Could you check a few things on this model? Use its own coordinates, in mm. Face numbers are marked on the shaded views. A direction names the side the tool comes from. Coordinates: 2 decimals unless noted, no trailing zeros. Write each loop counter-clockwise with the first axis right and the second up, starting at its lowest first coordinate (ties: lowest second). Pieces come first, ordered by that corner, then holes.
Item 1: I want a section at C-C on z = 3. Please give me the cut outline in (x, y).
Item 2: Which directions (+Z, -Z, +X, -X, +Y, -Y) give clear straight access to the entire face, cutting with the end or side of a thin tool? Please do the marked faces 5, 6 and 7.
Item 3: If I drill on probe 1 along X at (y, z) = (2, 10); probe 2 along X at (y, z) = (10, -14); probe 3 along X at (y, z) = (8, -11.5), over which ranges is the centre line in solid material (lowest first)?
Item 4: I want a section at A-A on x = 34.5. Please give me the cut outline in (y, z).
Item 5: Thinking about a two-plate mould opening in X: for the marked faces 1, 2, 3 and 4, which applies, +X half, -X half, draft (parallel to the pull), parting line (faces both ways), or undercut?
Item 6: For P1, Ø7, axis at x = 31.6, y = 4, coming from the -Z side, with a flat end and sliding along its axis, tell me the tip position at first contact or that it passes through.
Item 7: I want a section at B-B on z = -7. Please give me the cut outline in (x, y).
Item 8: I want a section at D-D on x = 6. Please give me the cut outline in (y, z).
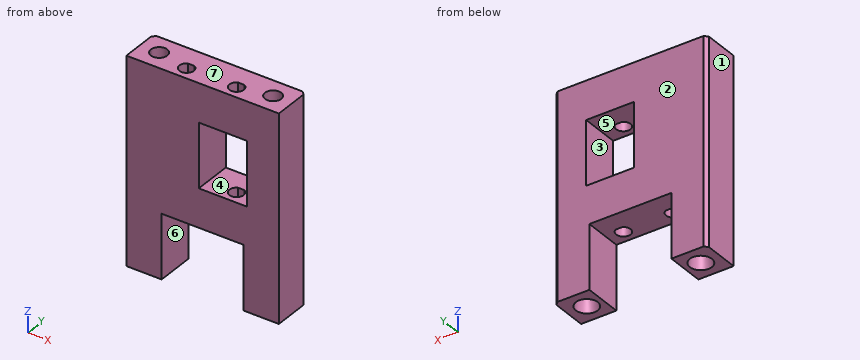
from build123d import *
from OCP.BRepFilletAPI import BRepFilletAPI_MakeChamfer

# Parameters (mm, degrees)
BOSS_EXTRUDE1_DEPTH = 44
SKETCH2_R           = 2.25
CUT_EXTRUDE1_DEPTH  = 66.098079849
BOSS_EXTRUDE2_START = 20
BOSS_EXTRUDE2_DEPTH = 20
BOSS_EXTRUDE3_START = -64
BOSS_EXTRUDE3_DEPTH = 64
SKETCH6_W           = 25.6
SKETCH6_H           = 20
CUT_EXTRUDE2_DEPTH  = 66.098079849
CHAMFER1_SIZE       = 10
CHAMFER1_SIZE2      = 0.874886635
CHAMFER2_SIZE       = 1
SKETCH7_W           = 15
SKETCH7_H           = 20
CUT_EXTRUDE3_DEPTH  = 66.922378598


with BuildPart() as part:
    # Sketch1 → Boss-Extrude1 (new body)
    with BuildSketch(Plane.XY):
        with BuildLine():
            Line((0, 0), (47.6, 0))
            Line((47.6, 0), (47.6, 6))
            Line((47.6, 6), (44.15, 6))
            ThreePointArc((44.15, 6), (41.6, 3.45), (39.05, 6))
            Line((39.05, 6), (8.55, 6))
            ThreePointArc((8.55, 6), (6, 3.45), (3.45, 6))
            Line((3.45, 6), (0, 6))
            Line((0, 6), (0, 0))
        make_face()
    extrude(amount=BOSS_EXTRUDE1_DEPTH)

    # Sketch2 → Cut-Extrude1 (cut, through all)
    with BuildSketch(Plane.XY.offset(44)):
        with Locations((16, 4)):
            Circle(SKETCH2_R)
        with Locations((31.6, 4)):
            Circle(SKETCH2_R)
    extrude(amount=-CUT_EXTRUDE1_DEPTH, mode=Mode.SUBTRACT)

    # Sketch4 → Boss-Extrude2 (add)
    with BuildSketch(Plane(origin=(0, 0, 0), x_dir=(-1, 0, 0), z_dir=(0, 0, -1)).offset(BOSS_EXTRUDE2_START)):
        with BuildLine():
            Line((-11, 6), (-11, 0))
            Line((-11, 0), (0, 0))
            Line((0, 0), (0, 6))
            Line((0, 6), (-3.45, 6))
            ThreePointArc((-3.45, 6), (-6, 3.45), (-8.55, 6))
            Line((-8.55, 6), (-11, 6))
        make_face()
        with BuildLine():
            Line((-36.6, 6), (-36.6, 0))
            Line((-36.6, 0), (-47.6, 0))
            Line((-47.6, 0), (-47.6, 6))
            Line((-47.6, 6), (-44.15, 6))
            ThreePointArc((-44.15, 6), (-41.6, 3.45), (-39.05, 6))
            Line((-39.05, 6), (-36.6, 6))
        make_face()
    extrude(amount=-BOSS_EXTRUDE2_DEPTH)

    # Sketch5 → Boss-Extrude3 (add)
    with BuildSketch(Plane.XY.offset(44).offset(BOSS_EXTRUDE3_START)):
        with BuildLine():
            Line((0, 6), (0, 12))
            Line((0, 12), (47.6, 12))
            Line((47.6, 12), (47.6, 6))
            Line((47.6, 6), (44.15, 6))
            ThreePointArc((44.15, 6), (41.6, 8.55), (39.05, 6))
            Line((39.05, 6), (8.55, 6))
            ThreePointArc((8.55, 6), (6, 8.55), (3.45, 6))
            Line((3.45, 6), (0, 6))
        make_face()
    extrude(amount=BOSS_EXTRUDE3_DEPTH)

    # Sketch6 → Cut-Extrude2 (cut, through all)
    with BuildSketch(Plane.XZ.offset(-6)):
        with Locations((23.8, -10)):
            Rectangle(SKETCH6_W, SKETCH6_H)
    extrude(amount=-CUT_EXTRUDE2_DEPTH, mode=Mode.SUBTRACT)

    # Chamfer1: one chamfer whose edges measure the first distance from different faces: ONE call of the kernel's chamfer builder (chamfer() names one face for all edges)
    chamfer1_edges_1 = [part.edges().sort_by_distance(p)[0] for p in [
        (6, 3.45, -20),
    ]]
    chamfer1_side_1 = [part.faces().sort_by_distance(p)[0] for p in [
        (6, 3.45, 12),
    ]]
    chamfer1_edges_2 = [part.edges().sort_by_distance(p)[0] for p in [
        (41.6, 8.55, -20),
    ]]
    chamfer1_side_2 = [part.faces().sort_by_distance(p)[0] for p in [
        (41.6, 8.55, 12),
    ]]
    chamfer1 = BRepFilletAPI_MakeChamfer(part.part.solid().wrapped)
    for e in chamfer1_edges_1:
        chamfer1.Add(CHAMFER1_SIZE, CHAMFER1_SIZE2, e.wrapped, chamfer1_side_1[0].wrapped)  # the first distance lies on this face
    for e in chamfer1_edges_2:
        chamfer1.Add(CHAMFER1_SIZE, CHAMFER1_SIZE2, e.wrapped, chamfer1_side_2[0].wrapped)  # the first distance lies on this face
    add(Compound.cast(chamfer1.Shape()), mode=Mode.REPLACE)

    # Chamfer2
    chamfer2_edges = [part.edges().sort_by_distance(p)[0] for p in [
        (47.6, 12, 12),
        (0, 12, 12),
    ]]
    chamfer(chamfer2_edges, length=CHAMFER2_SIZE)

    # Sketch7 → Cut-Extrude3 (cut, through all)
    with BuildSketch(Plane.XZ):
        with Locations((30.1, 22)):
            Rectangle(SKETCH7_W, SKETCH7_H)
    extrude(amount=-CUT_EXTRUDE3_DEPTH, mode=Mode.SUBTRACT)


solid = part.part
Response values:
1. outline: (0, 0) - (47.6, 0) - (47.6, 11) - (46.6, 12) - (1, 12) - (0, 11) - close; hole circle Ø5.1 at (6, 6); hole (14.97, 6) arc R2.25 ccw (long way) to (17.03, 6) - close; hole (30.57, 6) arc R2.25 ccw (long way) to (32.63, 6) - close; hole circle Ø5.1 at (41.6, 6)
2. face 5: +Y, -Y
2. face 6: -Z, +Y, -Y
2. face 7: +Z, +X, -X, +Y, -Y
3. probe 1: x = 0 to 14.97, 17.03 to 30.57, 32.63 to 47.6
3. probe 2: x = 0 to 11, 36.6 to 47.6
3. probe 3: x = 0 to 4.21, 7.79 to 11, 36.6 to 39.81, 43.39 to 47.6
4. outline: (0, 0) - (12, 0) - (12, 12) - (0, 12) - close; (0, 32) - (12, 32) - (12, 44) - (0, 44) - close
5. face 1: -X half
5. face 2: draft
5. face 3: undercut
5. face 4: undercut
6. P1: stops at z = 0
7. outline: (0, 0) - (11, 0) - (11, 12) - (1, 12) - (0, 11) - close; (36.6, 0) - (47.6, 0) - (47.6, 11) - (46.6, 12) - (36.6, 12) - close; hole circle Ø5.1 at (6, 6); hole circle Ø5.1 at (41.6, 6)
8. outline: (0, -20) - (2.58, -20) - (3.45, -10) - (3.45, 44) - (0, 44) - close; (8.55, -10) - (9.42, -20) - (12, -20) - (12, 44) - (8.55, 44) - close
